The model under review builds one solid part; all positions refer to its coordinate system, in mm. Round coordinates to 2 decimals unless told otherwise and drop trailing zeros. Loops run counter-clockwise (first coordinate to the right, second up) from the corner with the lowest first, then second, coordinate; pieces in that order, holes last. Notation, with made-up numbers: M 6,68.25 L 48,68.25 A32 ccw 48,95.25 Z; hole C -3,31 d5. An arc over 180 degrees is marked long. Use a Markdown table: item, result. Add a question column.
Autodesk Fusion 360 part; units mm, degrees
sketch "Sketch1" plane through (0, 0, 0) normal (0, 0, 1) x (1, 0, 0)
  line L0 (0, 0) -> (342.375, 0)
  line L1 (342.375, 0) -> (342.375, 123.3)
  line L2 (342.375, 123.3) -> (0, 123.3)
  line L3 (0, 123.3) -> (0, 0)
  dimension "d1" = 342.375
  dimension "d2" = 123.3
extrude "Extrude1" add sketch "Sketch1" along normal blind 1
fillet "Fillet1" radius 2.5 4 edges at (0, 0, 0.5) (342.375, 0, 0.5) (342.375, 123.3, 0.5) (0, 123.3, 0.5)
sketch "Sketch2" plane through (0, 0, 1) normal (0, 0, 1) x (-1, 0, 0)
  arc A0 (-2.5, -123.3) -> (0, -120.8) centre (-2.5, -120.8) ccw
  line L0 (0, -120.8) -> (0, -2.5)
  arc A1 (0, -2.5) -> (-2.5, 0) centre (-2.5, -2.5) ccw
  line L1 (-2.5, 0) -> (-339.875, 0)
  arc A2 (-339.875, 0) -> (-342.375, -2.5) centre (-339.875, -2.5) ccw
  line L2 (-342.375, -2.5) -> (-342.375, -120.8)
  arc A3 (-342.375, -120.8) -> (-339.875, -123.3) centre (-339.875, -120.8) ccw
  line L3 (-339.875, -123.3) -> (-2.5, -123.3)
  line L4 (-5.5, -117.8) -> (-5.5, -5.5) construction
  line L5 (-5.5, -5.5) -> (-336.147, -5.5) construction
  line L6 (-5.5, -117.8) -> (-336.856, -117.8) construction
  line L7 (-336.147, -5.5) -> (-336.856, -117.8) construction
  line L8 (-336.147, -5.5) -> (-5.5, -117.8)
  line L9 (-5.5, -5.5) -> (-336.856, -117.8)
  line L10 (-5.9, -117.1907) -> (-5.9, -117.4)
  line L11 (-7.5002, -117.4) -> (-5.9, -117.4)
  line L12 (-8, -5.9) -> (-5.9, -5.9)
  line L13 (-5.9, -117.1907) -> (-5.9, -5.9)
  line L14 (-5.9, 0) -> (-5.9, 15)
  line L15 (-7.5002, -117.4) -> (-335.747, -117.4)
  line L16 (-8, -5.9) -> (-335.747, -5.9)
  line L17 (-335.747, -5.9) -> (-335.747, -117.4242)
  dimension "d7" = 5.5
  dimension "d8" = 5.5
  dimension "d9" = 5.5
  dimension "d10" = 6.228
  dimension "d11" = 5.519
  dimension "d16" = 0.4
  dimension "d17" = 0.4
  dimension "d18" = 0.4
extrude "Extrude2" add sketch "Sketch2" along normal blind 2 contours L8 L9 L12 L16 | L8 L9 L15 L16 L17 | L8 L9 L10 L11 L12 L13 | L8 L9 L11 L15
sketch "Sketch3" plane through (0, 0, 1) normal (0, 0, 1) x (-1, 0, 0)
  line L0 (-5.9, -5.9) -> (-5.9, -117.4)
  line L1 (-5.9, -117.4) -> (-335.747, -117.4)
  line L2 (-335.747, -117.4) -> (-335.747, -5.9)
  line L3 (-335.747, -5.9) -> (-5.9, -5.9)
  arc A0 (-2.5, -123.3) -> (0, -120.8) centre (-2.5, -120.8) ccw
  line L4 (0, -120.8) -> (0, -2.5)
  arc A1 (0, -2.5) -> (-2.5, 0) centre (-2.5, -2.5) ccw
  line L5 (-2.5, 0) -> (-339.875, 0)
  arc A2 (-339.875, 0) -> (-342.375, -2.5) centre (-339.875, -2.5) ccw
  line L6 (-342.375, -2.5) -> (-342.375, -120.8)
  arc A3 (-342.375, -120.8) -> (-339.875, -123.3) centre (-339.875, -120.8) ccw
  line L7 (-339.875, -123.3) -> (-2.5, -123.3)
  line L8 (-6.2203, -99.9759) -> (-6.2199, -118.8)
  line L9 (-6.2246, -4.5) -> (-6.2082, -61.8661)
  line L10 (-6.2082, -61.8661) -> (-6.2095, -61.8663)
  line L11 (0.0269, -120.8) -> (-0.7247, -2.5)
  line L12 (-125.03, -5.5) -> (-14.265, -5.5)
  line L13 (-14.2649, -117.8) -> (-73.858, -117.8)
  line L14 (-14.265, -4.5) -> (-6.2246, -4.5)
  line L15 (-14.265, -5.5) -> (-6.2247, -5.5)
  line L16 (-14.2649, -117.8004) -> (-6.2199, -117.8002)
  arc A4 (-2.4783, -123.3004) -> (0.0269, -120.8) centre (-2.459, -120.8147) ccw
  line L17 (-6.2095, -61.8663) -> (-6.2054, -78.9217)
  line L18 (-133.07, -5.5) -> (-133.07, -4.5)
  line L19 (-73.858, -117.8) -> (-73.858, -118.8)
  line L20 (-81.898, -118.8) -> (-81.898, -117.8)
  arc A5 (-0.7247, -2.5) -> (-3.225, 0) centre (-3.2248, -2.5001) ccw
  line L21 (-332.837, -117.8) -> (-333.8375, -117.8)
  line L22 (-332.8375, -4) -> (-332.8375, -2.5)
  line L23 (-332.837, -4) -> (-310.8413, -4)
  line L24 (-73.858, -117.8003) -> (-73.858, -118.8)
  line L25 (-73.858, -118.8) -> (-81.898, -118.8)
  line L26 (-340.62, -123.2958) -> (-335.838, -123.3)
  line L27 (-81.898, -118.8) -> (-81.898, -117.8)
  line L28 (-332.837, -118.8) -> (-332.837, -117.8)
  line L29 (-333.8375, -118.8) -> (-333.838, -118.8)
  arc A6 (-343.1178, -120.7937) -> (-340.62, -123.2958) centre (-340.6178, -120.7958) ccw
  line L30 (-247.164, -117.8) -> (-324.797, -117.8)
  line L31 (-296.48, -4.5) -> (-296.48, -5.5)
  line L32 (-333.8375, -117.8) -> (-333.8375, -118.8)
  line L33 (-337.5995, -117.8) -> (-337.5995, -4)
  line L34 (-333.838, -117.8) -> (-337.5995, -117.8)
  line L35 (-247.164, -118.8) -> (-247.164, -117.8)
  line L36 (-324.797, -118.8) -> (-332.837, -118.8)
  line L37 (-333.838, -118.8) -> (-333.838, -117.8)
  line L38 (-324.797, -117.8) -> (-324.797, -118.8)
  line L39 (-3.225, 0) -> (-340.5995, 0)
  line L40 (-343.0995, -99.75) -> (-343.1178, -120.7937)
  line L41 (-6.2083, -80.9225) -> (-6.2049, -97.9745)
  line L42 (-6.2062, -99.9739) -> (-6.2203, -99.9759)
  line L43 (-6.2065, -80.9222) -> (-6.2083, -80.9225)
  line L44 (-310.8413, -4) -> (-310.8413, -5.5)
  line L45 (-343.0995, -2.5) -> (-343.0995, -99.75)
  arc A7 (-0.7247, -2.5) -> (-3.225, 0.0001) centre (-3.2248, -2.5001) ccw
  line L46 (-6.2054, -78.9217) -> (-6.207, -78.922)
  line L47 (-332.837, -2.5) -> (-332.837, -4)
  line L48 (-337.5995, -4) -> (-332.8375, -4)
  line L49 (-304.52, -5.5) -> (-304.52, -4.5)
  arc A8 (-340.5995, 0) -> (-343.0995, -2.5) centre (-340.5995, -2.5) ccw
  line L50 (-335.838, -123.3) -> (-2.4783, -123.3004)
  line L51 (-310.8413, -5.5) -> (-304.52, -5.5)
  line L52 (-6.2083, -61.8661) -> (-6.2095, -61.8663)
  line L53 (-304.52, -4.5) -> (-296.48, -4.5)
  line L54 (-296.48, -5.5) -> (-133.07, -5.5)
  line L55 (-332.8375, -2.5) -> (-332.837, -2.5)
  line L56 (-14.265, -5.5) -> (-14.265, -4.5)
  line L57 (-14.265, -4.5) -> (-6.225, -4.5)
  line L58 (-6.2095, -61.8663) -> (-6.2054, -78.9217)
  line L59 (-6.225, -4.5) -> (-6.2083, -61.8661)
  line L60 (-81.898, -117.8) -> (-239.124, -117.8)
  line L61 (-337.5995, -117.8) -> (-337.5995, -4)
  line L62 (-3.225, 0.0001) -> (-340.5995, 0)
  line L63 (-335.838, -123.3) -> (-2.4783, -123.3)
  line L64 (-247.164, -117.8) -> (-324.797, -117.8)
  line L65 (-296.48, -5.5) -> (-133.07, -5.5)
  line L66 (-14.2649, -117.8004) -> (-73.858, -117.8003)
  line L67 (-6.2203, -99.9759) -> (-6.2199, -118.8)
  line L68 (-6.2065, -80.9222) -> (-6.2083, -80.9225)
  line L69 (-6.207, -78.922) -> (-6.2065, -80.9222)
  line L70 (-6.2083, -80.9225) -> (-6.2049, -97.9745)
  line L71 (-6.2049, -97.9745) -> (-6.2066, -97.9748)
  line L72 (-6.2066, -97.9748) -> (-6.2062, -99.9739)
  line L73 (-14.2649, -118.8) -> (-14.2649, -117.8004)
  arc A9 (-2.4783, -123.3) -> (0.0217, -120.8) centre (-2.4626, -120.8157) ccw
  line L74 (-125.03, -5.5) -> (-14.265, -5.5)
  line L75 (-6.2199, -118.8) -> (-14.2649, -118.8)
  line L76 (0.0217, -120.8) -> (-0.7247, -2.5)
  line L77 (-6.2062, -99.9739) -> (-6.2203, -99.9759)
  line L78 (-247.164, -118.8) -> (-247.164, -117.8)
  line L79 (-239.124, -118.8) -> (-247.164, -118.8)
  line L80 (-333.838, -118.8) -> (-333.838, -117.8)
  line L81 (-310.8413, -4) -> (-310.8413, -5.5)
  line L82 (-333.8375, -118.8) -> (-333.838, -118.8)
  line L83 (-333.8375, -117.8) -> (-333.8375, -118.8)
  line L84 (-332.8375, -4) -> (-332.8375, -2.5)
  line L85 (-332.837, -4) -> (-310.8413, -4)
  line L86 (-332.837, -117.8) -> (-333.8375, -117.8)
  line L87 (-332.837, -118.8) -> (-332.837, -117.8)
  line L88 (-332.8375, -2.5) -> (-332.837, -2.5)
  line L89 (-324.797, -118.8) -> (-332.837, -118.8)
  line L90 (-239.124, -117.8) -> (-239.124, -118.8)
  line L91 (-324.797, -117.8) -> (-324.797, -118.8)
  line L92 (-333.838, -117.8) -> (-337.5995, -117.8)
  line L93 (-296.48, -4.5) -> (-296.48, -5.5)
  line L94 (-332.837, -2.5) -> (-332.837, -4)
  arc A10 (-343.1178, -120.7937) -> (-340.62, -123.2958) centre (-340.6178, -120.7958) ccw
  line L95 (-343.0995, -99.75) -> (-343.1178, -120.7937)
  line L96 (-343.0995, -2.5) -> (-343.0995, -99.75)
  line L97 (-304.52, -5.5) -> (-304.52, -4.5)
  line L98 (-337.5995, -4) -> (-332.8375, -4)
  line L99 (-310.8413, -5.5) -> (-304.52, -5.5)
  arc A11 (-340.5995, 0) -> (-343.0995, -2.5) centre (-340.5995, -2.5) ccw
  line L100 (-304.52, -4.5) -> (-296.48, -4.5)
  line L101 (-340.62, -123.2958) -> (-335.838, -123.3)
  line L102 (-6.2066, -97.9748) -> (-6.2062, -99.9739)
  line L103 (-6.2199, -118.8) -> (-14.2649, -118.8)
  line L104 (-14.2649, -118.8) -> (-14.2649, -117.8)
  line L105 (-6.2049, -97.9745) -> (-6.2066, -97.9748)
  line L106 (-6.207, -78.922) -> (-6.2065, -80.9222)
  line L107 (-6.2054, -78.9217) -> (-6.207, -78.922)
  line L108 (-14.265, -5.5) -> (-14.265, -4.5)
  line L109 (-125.03, -4.5) -> (-125.03, -5.5)
  line L110 (-73.858, -118.8) -> (-81.898, -118.8)
  line L111 (-125.03, -4.5) -> (-125.03, -5.5)
  line L112 (-133.07, -4.5) -> (-125.03, -4.5)
  line L113 (-81.898, -117.8) -> (-239.124, -117.8)
  line L114 (-239.124, -117.8) -> (-239.124, -118.8)
  line L115 (-239.124, -118.8) -> (-247.164, -118.8)
  line L116 (-133.07, -5.5) -> (-133.07, -4.5)
  line L117 (-133.07, -4.5) -> (-125.03, -4.5)
  point P0 (-304.5, -5.5)
  dimension "d22" = 5.5
  dimension "d23" = 5.5
  dimension "d24" = 6.2339
  dimension "d25" = 5.5125
  dimension "d26" = 5.5
  dimension "d27" = 6.2276
  dimension "d28" = 5.5188
equation "d1 = 337.375 mm + 2.5 mm + 2.5 mm"
equation "d2 = 118.3 mm + 2.5 mm + 2.5 mm"
(1) Consider section C-C, the plane z = 2.05. Give the boundary of the cut face in (x, y), then the cut area to 3 significant figures.
(2) Insertion check: pin 1 Ø0.6 at (y, z) = (39.5, 1.5) entering from -X; pin 2 Ø5 at (x, y) = (229, 37) entering from -Z; pin 3 Ø0.6 at (y, z) = (59.5, 2) entering from +X; pin 4 Ø1 at (x, z) = (141, 2.5) entering from -Y. Each pin has a flat end and moves straight along its axis. Give the tip position at first contact, or say it passes through.
(3) To check wall thickness, follow probe 1 along X at (y, z) = (39, 2.2); probe 2 along Y at (x, z) = (205, 2); probe 3 along Z at (x, y) = (309.5, 118). State the ranges of each line that lie inside material, in increasing order.
(4) Consider section A-A, the plane y = 54. Give the boundary of the cut face in (x, z) (3 decimals), then the cut area to 3 significant figures.
(5) Consider section B-B, the plane x = 197. Give the boundary of the cut face in (y, z), then the cut area to 3 significant figures.
Found:
| question | item | result |
|---|---|---|
| 1 | outline | M 5.9,5.9 L 335.75,5.9 L 335.75,117.4 L 5.9,117.4 Z |
| 1 | area | 36,800 mm^2 |
| 2 | pin 1 | stops at x = 5.9 |
| 2 | pin 2 | stops at z = 0 |
| 2 | pin 3 | stops at x = 335.75 |
| 2 | pin 4 | stops at y = 5.9 |
| 3 | probe 1 | x = 5.9 to 335.75 |
| 3 | probe 2 | y = 5.9 to 117.4 |
| 3 | probe 3 | z = 0 to 1 |
| 4 | outline | M 0,0 L 342.375,0 L 342.375,1 L 335.747,1 L 335.747,3 L 5.9,3 L 5.9,1 L 0,1 Z |
| 4 | area | 1,000 mm^2 |
| 5 | outline | M 0,0 L 123.3,0 L 123.3,1 L 117.4,1 L 117.4,3 L 5.9,3 L 5.9,1 L 0,1 Z |
| 5 | area | 346 mm^2 |
